```python
from build123d import *

# Parameters (mm, degrees)
ESQUISSE2_R             = 2
ENL_V_MAT_EXTRU_1_DEPTH = 12.5


with BuildPart() as part:
    # Esquisse1 → Base-R_volution (revolve)
    with BuildSketch(Plane.XY, mode=Mode.PRIVATE) as base_r_volution_sk:
        Polygon((-0.5, 8), (0, 7.5), (0, 5), (-50, 5), (-50, 7.5), (-49.5, 8), align=None)
    revolve(base_r_volution_sk.sketch.rotate(Axis((-22.885527638, 0, 0), (1, 0, 0)), 90), axis=Axis((-22.885527638, 0, 0), (1, 0, 0)))

    # Esquisse2 → Enl_v. mat.-Extru.1 (cut, symmetric)
    with BuildSketch(Plane.XY):
        with Locations((-38, 0)):
            Circle(ESQUISSE2_R)
    extrude(amount=ENL_V_MAT_EXTRU_1_DEPTH, both=True, mode=Mode.SUBTRACT)


solid = part.part
```
Verification items for the finished model (mm, model axes). Coordinates: 2 decimals unless noted, no trailing zeros. Write each loop counter-clockwise with the first axis right and the second up, starting at its lowest first coordinate (ties: lowest second). Pieces come first, ordered by that corner, then holes. Notation, with made-up numbers: M -8,-37 L 38,-37 A28 cw 38,-13 Z; hole C 64,86.5 d10. An arc over 180 degrees is marked long. Answer as a JSON object with one key per item and string values. Group by question number.
(1) Cross-section at B-B, the plane z = 0. Record the cut outline in (x, y), and give its area (4 significant figures).
(2) Cross-section at D-D, the plane x = -16.5. Record the cut outline in (y, z), and give its area (3 significant figures).
(3) Cross-section at A-A, the plane y = 0. Record the cut outline in (x, z).
(4) Release check for a two-part mould opening along Y. For faces 1 (the face through (-25.35, -1.5, 4.77)), 2 (the face through (-24.66, 7.81, -1.73)), 3 (the face through (0, 5, 2)) record: +Y half, -Y half, draft (parallel to the pull), parting line (faces both ways), or undercut.
(5) Cross-section at C-C, the plane x = -38. Record the cut outline in (y, z), and give its area (3 significant figures).
(6) Gauge pin test, flat end, axial feed: pin 1 (1.5 mm diameter, centred on x = -13, z = 3.5, fed in from -Y). Record the tip position at first contact, or that the pin passes through.
(7) Material ranges on line 1 (Y direction, x = -10, z = -0.5); line 2 (Z direction, x = -17, y = -0.75); line 3 (Y direction, x = -38, z = -6.3), recorded low to high.
Reply:
{
 "1": {"outline": "M -50,-7.5 L -49.5,-8 L -0.5,-8 L 0,-7.5 L 0,-5 L -50,-5 Z; M -50,5 L 0,5 L 0,7.5 L -0.5,8 L -49.5,8 L -50,7.5 Z", "area": "299.5 mm²"},
 "2": {"outline": "C 0,0 d16; hole C 0,0 d10", "area": "123 mm²"},
 "3": {"outline": "M -50,-7.5 L -49.5,-8 L -40,-8 L -40,-5 L -50,-5 Z; M -50,5 L -40,5 L -40,8 L -49.5,8 L -50,7.5 Z; M -36,-8 L -0.5,-8 L 0,-7.5 L 0,-5 L -36,-5 Z; M -36,5 L 0,5 L 0,7.5 L -0.5,8 L -36,8 Z"},
 "4": {"face 1": "undercut", "face 2": "parting line", "face 3": "draft"},
 "5": {"outline": "M -2,-7.75 L -2,-4.58 A5 cw -2,4.58 L -2,7.75 A8 ccw Z; M 2,-7.75 A8 ccw 2,7.75 L 2,4.58 A5 cw 2,-4.58 Z", "area": "98.1 mm²"},
 "6": {"pin 1": "y = -7.51"},
 "7": {"line 1": "-7.98 to -4.97, 4.97 to 7.98", "line 2": "-7.96 to -4.94, 4.94 to 7.96", "line 3": "-4.93 to -2, 2 to 4.93"}
}
